Geometry: see drawing. Coordinates: mm, zero at the bounding-box minimum. A direction names the side the tool comes from. Coordinates: 2 decimals unless noted, no trailing zeros. Order: outer loops, then holes, each group sorted by start corner. A loop starts at its lowest first (then second) coordinate and runs counter-clockwise, first axis right, second up.
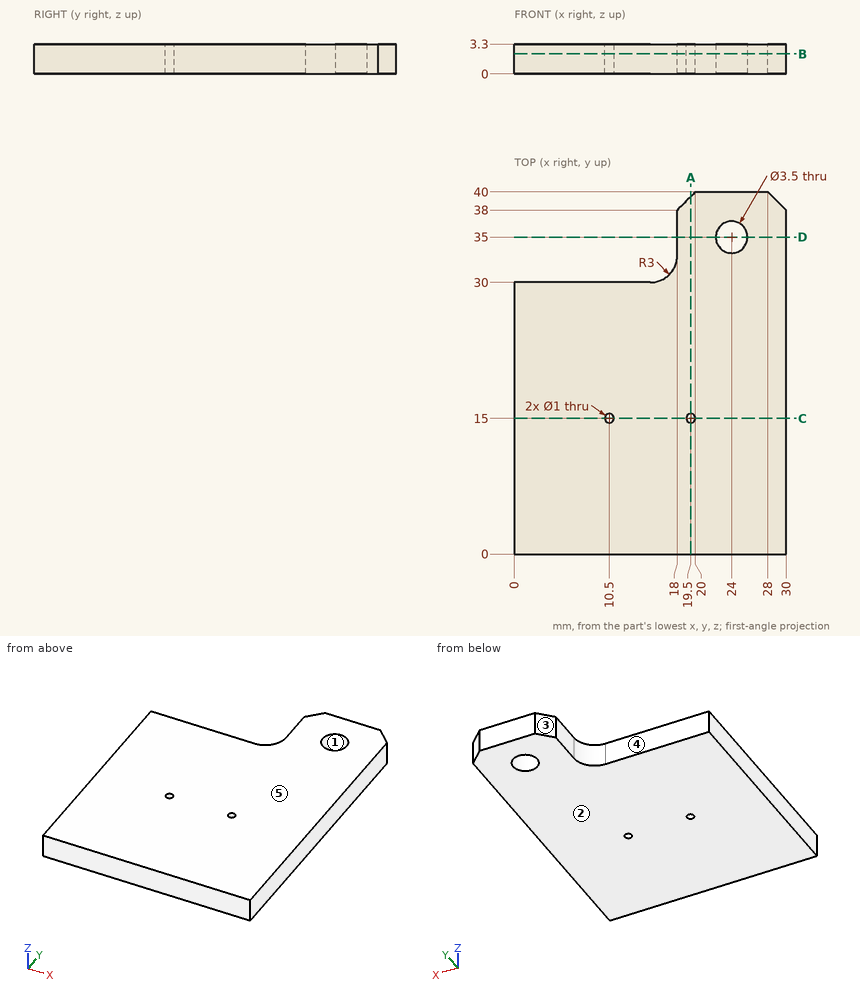
Item 1: Pin query (flat end, axial travel): pin 1 Ø2 at (x, y) = (24, 35) entering from -Z; pin 2 Ø1.6 at (x, z) = (7, 1) entering from +Y. Return the tip coordinate at first contact, or that it passes through.
Response values:
pin 1: passes through
pin 2: stops at y = 30
Item 2: Cut plane D-D on y = 35. Return loops of the section in (x, z).
Response values:
outline: (18, 0) - (22.25, 0) - (22.25, 3.3) - (18, 3.3) - close; (25.75, 0) - (30, 0) - (30, 3.3) - (25.75, 3.3) - close
Item 3: Cut plane B-B on z = 2.2. Return loops of the section in (x, y).
Response values:
outline: (0, 0) - (30, 0) - (30, 38) - (28, 40) - (20, 40) - (18, 38) - (18, 33) arc R3 cw to (15, 30) - (0, 30) - close; hole circle Ø1 at (10.5, 15); hole circle Ø1 at (19.5, 15); hole circle Ø3.5 at (24, 35)
Item 4: Ray query, probe 1 along Y at (x, z) = (24, 1.8); probe 2 along Y at (x, z) = (6.75, 0.7); probe 3 along Y at (x, z) = (10.5, 1.1). Return the intervals inside material, ascending.
Response values:
probe 1: y = 0 to 33.25, 36.75 to 40
probe 2: y = 0 to 30
probe 3: y = 0 to 14.5, 15.5 to 30
Item 5: Cut plane A-A on x = 19.5. Return loops of the section in (y, z).
Response values:
outline: (0, 0) - (14.5, 0) - (14.5, 3.3) - (0, 3.3) - close; (15.5, 0) - (39.5, 0) - (39.5, 3.3) - (15.5, 3.3) - close
Item 6: Draft query along X for the marked faces 1, 2 and 3. Return one class per face: pulls with the +X half, pulls with the -X half, needs draft (parallel to the pull), parting line crosses it, or undercut.
Response values:
face 1: undercut
face 2: needs draft
face 3: pulls with the -X half
Item 7: Access query for the marked faces 4 and 5. Directions: +Z, -Z, +X, -X, +Y, -Y. A direction counts if a zero-diameter tool reaches every point of the face in a straight line with its end or side. Return the directions, or none.
Response values:
face 4: +Z, -Z, -X, +Y
face 5: +Z, +X, -X, +Y, -Y
Item 8: Cut plane C-C on y = 15. Return loops of the section in (x, z).
Response values:
outline: (0, 0) - (10, 0) - (10, 3.3) - (0, 3.3) - close; (11, 0) - (19, 0) - (19, 3.3) - (11, 3.3) - close; (20, 0) - (30, 0) - (30, 3.3) - (20, 3.3) - close
